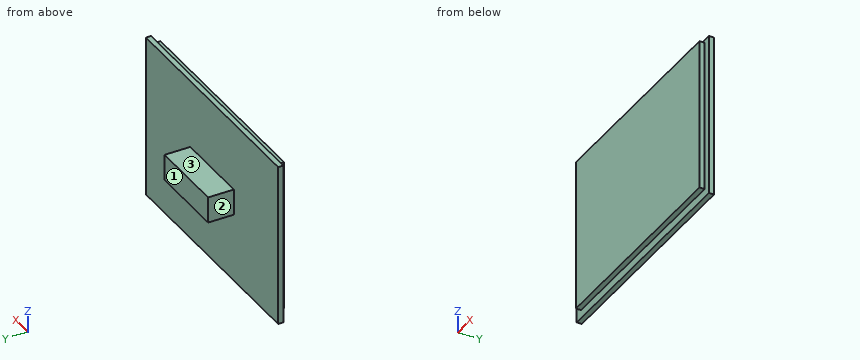
Autodesk Inventor part; units mm, degrees
ref_plane "YZ Plane" through (0, 0, 0) normal (1, 0, 0) x (0, 1, 0)
ref_plane "XZ Plane" through (0, 0, 0) normal (0, 1, 0) x (-1, 0, 0)
ref_plane "XY Plane" through (0, 0, 0) normal (0, 0, 1) x (1, 0, 0)
sketch "Sketch1" plane through (0, 0, 0) normal (0, 1, 0) x (-1, 0, 0)
  line L0 (0, 0) -> (-42.9, 0)
  line L1 (-42.9, 0) -> (-42.9, -29.75)
  line L2 (-42.9, -29.75) -> (0, -29.75)
  line L3 (0, -29.75) -> (0, 0)
  dimension "d0" = 42.9
  dimension "d1" = 29.75
extrude "Extrusion1" add sketch "Sketch1" along normal blind 1
sketch "Sketch2" plane through (0, 1, 0) normal (0, 1, 0) x (1, 0, 0)
  line L0 (42.9, 0) -> (42.9, 29.75)
  line L1 (42.9, 29.75) -> (0, 29.75)
  line L2 (-1.5, 31.392) -> (44.4, 31.392)
  line L3 (44.4, 31.392) -> (44.4, -0.507)
  line L4 (44.4, -0.507) -> (-1.5, -0.507)
  line L5 (-1.5, -0.507) -> (-1.5, 31.392)
  point P0 (0, 0)
extrude "Extrusion2" add sketch "Sketch2" along normal blind 1
sketch "Sketch3" plane through (0, 2, 0) normal (0, 1, 0) x (1, 0, 0)
  line L0 (-1.5, -0.507) -> (44.4, -0.507)
  line L1 (44.4, 31.392) -> (-1.5, 31.392)
  line L2 (-1.5, -0.507) -> (44.4, 31.392)
  line L3 (44.4, -0.507) -> (44.4, 31.392)
  line L4 (44.4, -0.507) -> (-1.5, 31.392)
  line L5 (13.9, 12.885) -> (29, 12.885)
  line L6 (29, 12.885) -> (29, 18)
  line L7 (29, 18) -> (13.9, 18)
  line L8 (13.9, 18) -> (13.9, 12.885)
  line L9 (13.9, 12.885) -> (29, 18) construction
  line L10 (29, 12.885) -> (13.9, 18) construction
  point P0 (0, 0)
  point P1 (21.45, 15.4425)
extrude "Extrusion3" add sketch "Sketch3" along normal blind 5 contours L5 L8 L7 L4 L2 | L2 L4 L5 | L4 L2 L7 L6 L5 | L4 L7 L2
properties part number "Lid"
The listing builds one solid part. Answer for the finished solid, in the listing's coordinates (mm). Face numbers are marked on the shaded views. A direction names the side the tool comes from. Coordinates: 2 decimals unless noted, no trailing zeros. Write each loop counter-clockwise with the first axis right and the second up, starting at its lowest first coordinate (ties: lowest second). Pieces come first, ordered by that corner, then holes. Notation, with made-up numbers: (26.25, 68.25) - (38.25, 68.25) arc R23 cw to (38.25, 106.25) - close; hole circle Ø9 at (16, -15.75). An arc over 180 degrees is marked (long way). One line per item, written item: value.
1) Find section C-C (y = 6). Give the vertices of the cut face in (x, z) (3 decimals).
Geometry check:
outline: (13.9, -18) - (29, -18) - (29, -12.885) - (13.9, -12.885) - close
2) Consider line 1 along X through (y, z) = (0.5, -5.5); line 2 along X through (y, z) = (2.25, -15); line 3 along Y through (x, z) = (32, -1). Determine where each line is inside the solid, lowest interval first. Write a range as from..to.
Geometry check:
line 1: x = 0..42.9
line 2: x = 13.9..29
line 3: y = 0..2
3) Find section B-B (x = 23). Give the vertices of the cut face in (y, z) (3 decimals), and give its area (3 significant figures).
Geometry check:
outline: (0, -29.75) - (1, -29.75) - (1, -31.392) - (2, -31.392) - (2, -18) - (7, -18) - (7, -12.885) - (2, -12.885) - (2, 0.507) - (1, 0.507) - (1, 0) - (0, 0) - close
area: 87.2 mm2
4) A tool of negligible diameter and unlimited length cuts with its end or side. For the marked faces 1, 2 and 3, from which of +Z, -Z, +X, -X, +Y, -Y can it reach the whole face along a straight path? Write none if from no direction.
Geometry check:
face 1: +Z, -Z, +X, -X, +Y
face 2: +Z, -Z, -X, +Y
face 3: +Z, +X, -X, +Y
5) Each of these flat-tipped pins is pushed along its axis until it touches: pin 1 Ø2.5 at (y, z) = (4, -14.5) entering from -X; pin 2 Ø4 at (x, y) = (21.5, 5.5) entering from -Z; pin 3 Ø3 at (y, z) = (4, -18) entering from +X. Where does it stop, or does it pass through?
Geometry check:
pin 1: stops at x = 13.9
pin 2: stops at z = -18
pin 3: stops at x = 29
6) Find section D-D (x = 39). Give the vertices of the cut face in (y, z).
Geometry check:
outline: (0, -29.75) - (1, -29.75) - (1, -31.39) - (2, -31.39) - (2, 0.51) - (1, 0.51) - (1, 0) - (0, 0) - close
7) Find section A-A (z = -6.5). Give the vertices of the cut face in (x, y).
Geometry check:
outline: (-1.5, 1) - (0, 1) - (0, 0) - (42.9, 0) - (42.9, 1) - (44.4, 1) - (44.4, 2) - (-1.5, 2) - close
